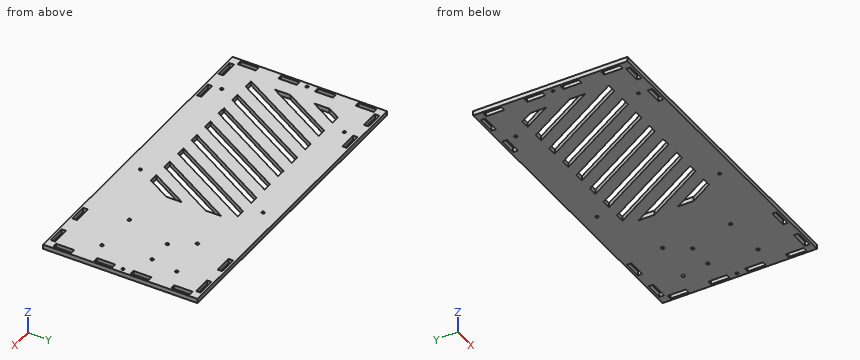
from build123d import *

# Parameters (mm, degrees)
F1_W     = 20
F1_H     = 5
F1_W_2   = 5
F1_H_2   = 20
F1_R     = 1.6
F1_R_2   = 1.75
F2_DEPTH = 5


with BuildPart() as f2:
    # F1 (on Top) → F2 (new body)
    with BuildSketch(Plane.XY):
        Polygon((0, 35), (0, 0), (350, 0), (350, 170), (0, 170), align=None)
        with Locations((20, 5)):
            Rectangle(F1_W, F1_H, mode=Mode.SUBTRACT)
        with Locations((5, 20)):
            Rectangle(F1_W_2, F1_H_2, mode=Mode.SUBTRACT)
        with Locations((60, 5)):
            Rectangle(F1_W, F1_H, mode=Mode.SUBTRACT)
        with Locations((49.5, 17.5)):
            Circle(F1_R, mode=Mode.SUBTRACT)
        with Locations((5, 65)):
            Rectangle(F1_W_2, F1_H_2, mode=Mode.SUBTRACT)
        with Locations((199.5, 17.5)):
            Circle(F1_R, mode=Mode.SUBTRACT)
        with Locations((290, 5)):
            Rectangle(F1_W, F1_H, mode=Mode.SUBTRACT)
        with Locations((330, 5)):
            Rectangle(F1_W, F1_H, mode=Mode.SUBTRACT)
        with Locations((345, 20)):
            Rectangle(F1_W_2, F1_H_2, mode=Mode.SUBTRACT)
        Polygon((209.5, 35), (199.5, 35), (224.5, 78.3012701892), (224.5, 60.9117498708), align=None, mode=Mode.SUBTRACT)
        Polygon((184.5, 35), (174.5, 35), (224.5, 121.6025403784), (224.5, 104.0979996554), align=None, mode=Mode.SUBTRACT)
        with Locations((274.1, 49.85)):
            Circle(F1_R_2, mode=Mode.SUBTRACT)
        with Locations((322.4, 48.45)):
            Circle(F1_R_2, mode=Mode.SUBTRACT)
        with Locations((345, 65)):
            Rectangle(F1_W_2, F1_H_2, mode=Mode.SUBTRACT)
        with Locations((5, 85)):
            Circle(F1_R, mode=Mode.SUBTRACT)
        with Locations((5, 105)):
            Rectangle(F1_W_2, F1_H_2, mode=Mode.SUBTRACT)
        Polygon((34.5, 35), (24.5, 35), (82.235026919, 135), (92.235026919, 135), align=None, mode=Mode.SUBTRACT)
        Polygon((59.5, 35), (49.5, 35), (107.235026919, 135), (117.235026919, 135), align=None, mode=Mode.SUBTRACT)
        Polygon((57.235026919, 135), (67.235026919, 135), (24.5, 60.9807621135), (24.5, 78.1862497847), align=None, mode=Mode.SUBTRACT)
        Polygon((32.235026919, 135), (42.235026919, 135), (24.5, 104.2820323028), (24.5, 121.3724995693), align=None, mode=Mode.SUBTRACT)
        Polygon((84.5, 35), (74.5, 35), (132.235026919, 135), (142.235026919, 135), align=None, mode=Mode.SUBTRACT)
        Polygon((109.5, 35), (99.5, 35), (157.235026919, 135), (167.235026919, 135), align=None, mode=Mode.SUBTRACT)
        Polygon((134.5, 35), (124.5, 35), (182.235026919, 135), (192.235026919, 135), align=None, mode=Mode.SUBTRACT)
        with Locations((5, 150)):
            Rectangle(F1_W_2, F1_H_2, mode=Mode.SUBTRACT)
        with Locations((20, 165)):
            Rectangle(F1_W, F1_H, mode=Mode.SUBTRACT)
        with Locations((49.5, 152.5)):
            Circle(F1_R, mode=Mode.SUBTRACT)
        with Locations((60, 165)):
            Rectangle(F1_W, F1_H, mode=Mode.SUBTRACT)
        Polygon((159.5, 35), (149.5, 35), (207.235026919, 135), (217.235026919, 135), align=None, mode=Mode.SUBTRACT)
        with Locations((289.3, 100.75)):
            Circle(F1_R_2, mode=Mode.SUBTRACT)
        with Locations((345, 85)):
            Circle(F1_R, mode=Mode.SUBTRACT)
        with Locations((317.5, 100.75)):
            Circle(F1_R_2, mode=Mode.SUBTRACT)
        with Locations((345, 105)):
            Rectangle(F1_W_2, F1_H_2, mode=Mode.SUBTRACT)
        with Locations((274.1, 124.75)):
            Circle(F1_R_2, mode=Mode.SUBTRACT)
        with Locations((199.5, 152.5)):
            Circle(F1_R, mode=Mode.SUBTRACT)
        with Locations((322.4, 130.75)):
            Circle(F1_R_2, mode=Mode.SUBTRACT)
        with Locations((290, 165)):
            Rectangle(F1_W, F1_H, mode=Mode.SUBTRACT)
        with Locations((345, 150)):
            Rectangle(F1_W_2, F1_H_2, mode=Mode.SUBTRACT)
        with Locations((330, 165)):
            Rectangle(F1_W, F1_H, mode=Mode.SUBTRACT)
    extrude(amount=F2_DEPTH)


solid = f2.part
The model under review builds one solid part; all positions refer to its coordinate system, in mm. Round coordinates to 2 decimals unless told otherwise and drop trailing zeros. Write item = value, one per line. Start each with the question number.
Item 1: To check wall thickness, follow L1, parallel to X at y = 20, z = 4.15; L2, parallel to Y at x = 336, z = 1.8; L3, parallel to X at y = 152.5, z = 2.7. State the ranges of each line that lie inside material, in increasing order.
Item 2: Take a section at A-A on z = 0.75. Count the separate pieces of the cut face and the enclosed holes in it, plus the area to 3 significant figures.
Item 3: Insertion check: pin 1 (1.5 mm diameter, centred on y = 5.5, z = 3, fed in from -X). The pin has a flat end and moves straight along its axis. Give the tip position at first contact, or say it passes through.
Result:
q1.L1 = 0 to 2.5, 7.5 to 342.5, 347.5 to 350
q1.L2 = 0 to 2.5, 7.5 to 162.5, 167.5 to 170
q1.L3 = 0 to 2.5, 7.5 to 47.9, 51.1 to 197.9, 201.1 to 342.5, 347.5 to 350
q2.separate_pieces = 1
q2.enclosed_holes = 38
q2.area = 49,800 mm²
q3.pin_1 = 0
